Build history of the part. All positions in model axes, mm. Round coordinates to 2 decimals unless told otherwise and drop trailing zeros. Loops run counter-clockwise (first coordinate to the right, second up) from the corner with the lowest first, then second, coordinate; pieces in that order, holes last. Notation, with made-up numbers: (65, 37.25) - (70, 37.25) arc R27 ccw to (70, 65.25) - close; hole circle Ø11 at (-20, 25.5). An arc over 180 degrees is marked (long way). Put each result on its own line as item: value. Start each with the question number.
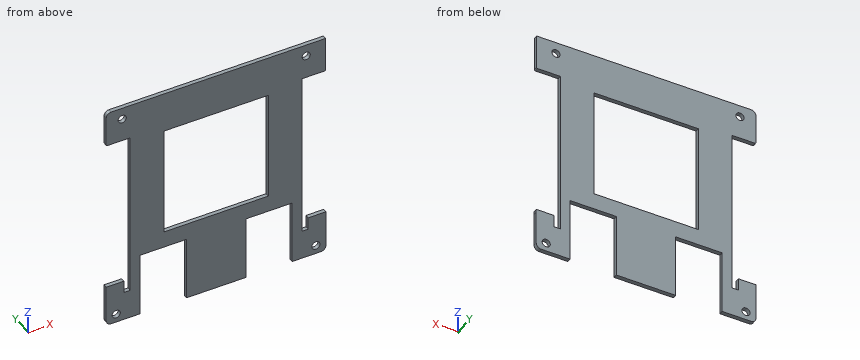
from build123d import *

# Parameters (mm, degrees)
SKETCH1_R                        = 1.6383
BOSS_EXTRUDE1_DEPTH              = 1.575
CUT_EXTRUDE1_DEPTH               = 2.54
CUTOUTS_FOR_THRUSTER_HEADS_DEPTH = 1.575
NOTCH_FOR_BPR_TOP_VIEW_W         = 2.575
NOTCH_FOR_BPR_TOP_VIEW_H         = 6.27
CUT_EXTRUDE11_DEPTH              = 10
NOTCH_FOR_BPL_TOP_VIEW_W         = 2.575
NOTCH_FOR_BPL_TOP_VIEW_H         = 6.27
CUT_EXTRUDE12_DEPTH              = 65.400936523
SKETCH22_W                       = 1.501374709
SKETCH22_H                       = 61.468
SKETCH22_W_2                     = 1.585
BOSS_EXTRUDE2_DEPTH              = 1.575
SKETCH23_W                       = 7.1002401
SKETCH23_H                       = 1.27
SKETCH23_W_2                     = 7.016
CUT_EXTRUDE13_DEPTH              = 65.400936523
SKETCH25_W                       = 2.5
SKETCH25_H                       = 44.79544
BOSS_EXTRUDE3_DEPTH              = 1.575
SKETCH26_W                       = 2.5
SKETCH26_H                       = 44.79544
BOSS_EXTRUDE4_DEPTH              = 1.575
SKETCH27_W                       = 41.818
SKETCH27_H                       = 1
CUT_EXTRUDE15_DEPTH              = 65.400936523
SKETCH28_W                       = 41.818
SKETCH28_H                       = 1
BOSS_EXTRUDE5_DEPTH              = 1.575


with BuildPart() as part:
    # Sketch1 → Boss-Extrude1 (new body)
    with BuildSketch(Plane(origin=(0, 0, 0), x_dir=(1, 0, 0), z_dir=(0, 1, 0))):
        with BuildLine():
            Line((-44, 45), (-44, 29.162404323))
            ThreePointArc((-44, 29.162404323), (-43.886381258, 28.888104416), (-43.612081351, 28.774485674))
            Line((-43.612081351, 28.774485674), (-33.211918649, 28.774485674))
            ThreePointArc((-33.211918649, 28.774485674), (-32.937618742, 28.660866933), (-32.824, 28.386567026))
            Line((-32.824, 28.386567026), (-32.824, -32.305595677))
            ThreePointArc((-32.824, -32.305595677), (-32.937618742, -32.579895584), (-33.211918649, -32.693514326))
            Line((-33.211918649, -32.693514326), (-36.100000052, -32.693514326))
            Line((-36.100000052, -32.693514326), (-43.612081299, -32.693514326))
            ThreePointArc((-43.612081299, -32.693514326), (-43.886381206, -32.807133067), (-43.999999948, -33.081432974))
            Line((-43.999999948, -33.081432974), (-43.999999948, -38.977))
            Line((-43.999999948, -38.977), (-43.999999948, -45))
            ThreePointArc((-43.999999948, -45), (-43.41421351, -46.414213562), (-41.999999948, -47))
            Line((-41.999999948, -47), (42.705916546, -47))
            Line((42.705916546, -47), (43.849731117, -47))
            Line((43.849731117, -47), (43.849731117, -38.27))
            Line((43.849731117, -38.27), (43.849731117, -33.081432974))
            ThreePointArc((43.849731117, -33.081432974), (43.736112376, -32.807133067), (43.461812469, -32.693514326))
            Line((43.461812469, -32.693514326), (36.098785193, -32.693514326))
            Line((36.098785193, -32.693514326), (33.824, -32.693514326))
            Line((33.824, -32.693514326), (32.822785141, -32.693514326))
            Line((32.822785141, -32.693514326), (32.822785141, -30.469351623))
            Line((32.822785141, -30.469351623), (32.822785141, 27.774485674))
            ThreePointArc((32.822785141, 27.774485674), (33.11567836, 28.481592456), (33.822785141, 28.774485674))
            Line((33.822785141, 28.774485674), (43.611054239, 28.774485674))
            ThreePointArc((43.611054239, 28.774485674), (43.885287743, 28.88803803), (43.998972842, 29.162216531))
            Line((43.998972842, 29.162216531), (44, 31.284))
            Line((44, 31.284), (44, 45))
            ThreePointArc((44, 45), (43.414213562, 46.414213562), (42, 47))
            Line((42, 47), (-42, 47))
            ThreePointArc((-42, 47), (-43.414213562, 46.414213562), (-44, 45))
        make_face()
        with Locations(Location((40, 43.5, 0), (0, 0, 270))):
            Circle(SKETCH1_R, mode=Mode.SUBTRACT)
        with Locations(Location((-40, 43.5, 0), (0, 0, 270))):
            Circle(SKETCH1_R, mode=Mode.SUBTRACT)
        with Locations(Location((-37.599999948, -42.2, 0), (0, 0, 270))):
            Circle(SKETCH1_R, mode=Mode.SUBTRACT)
        with Locations(Location((36.100000052, -42.2, 0), (0, 0, 270))):
            Circle(SKETCH1_R, mode=Mode.SUBTRACT)
        Polygon((23.409, -31.5), (-23.409, -31.5), (-23.409, 13.29544), (-12.909, 13.29544), (-12.909, 25.99544), (12.909, 25.99544), (12.909, 13.29544), (23.409, 13.29544), align=None, mode=Mode.SUBTRACT)
    extrude(amount=BOSS_EXTRUDE1_DEPTH)

    # Sketch2 → Cut-Extrude1 (cut)
    with BuildSketch(Plane(origin=(0, 1.575, 0), x_dir=(1, 0, 0), z_dir=(0, 1, 0))):
        Polygon((-12.909, 19.06), (-30.435, 19.06), (-30.435, 47), (30.435, 47), (30.435, 19.06), (12.909, 19.06), (12.909, 25.99544), (-12.909, 25.99544), align=None)
    extrude(amount=-CUT_EXTRUDE1_DEPTH, mode=Mode.SUBTRACT)

    # Sketch16 → Cutouts for Thruster Heads (add)
    with BuildSketch(Plane(origin=(0, 1.575, 0), x_dir=(1, 0, 0), z_dir=(0, 1, 0))):
        Polygon((12.909, 19.06), (12.909, 13.29544), (-12.909, 13.29544), (-12.909, 19.06), (-30.435, 19.06), (-30.435, 21), (-11.838888217, 21), (-11.838888217, 47), (11.909, 47), (11.909, 21), (30.435, 21), (30.435, 19.06), align=None)
    extrude(amount=-CUTOUTS_FOR_THRUSTER_HEADS_DEPTH)

    # Notch for BPR (TOP VIEW) → Cut-Extrude11 (cut)
    with BuildSketch(Plane(origin=(0, 1.575, 0), x_dir=(1, 0, 0), z_dir=(0, 1, 0))):
        with Locations((-35.6965, 31.909485674)):
            Rectangle(NOTCH_FOR_BPR_TOP_VIEW_W, NOTCH_FOR_BPR_TOP_VIEW_H)
    extrude(amount=-CUT_EXTRUDE11_DEPTH, mode=Mode.SUBTRACT)

    # Notch for BPL (TOP VIEW) → Cut-Extrude12 (cut, through all)
    with BuildSketch(Plane(origin=(0, 1.575, 0), x_dir=(1, 0, 0), z_dir=(0, 1, 0))):
        with Locations((35.61165985, 31.909485674)):
            Rectangle(NOTCH_FOR_BPL_TOP_VIEW_W, NOTCH_FOR_BPL_TOP_VIEW_H)
    extrude(amount=-CUT_EXTRUDE12_DEPTH, mode=Mode.SUBTRACT)

    # Sketch22 → Boss-Extrude2 (add)
    with BuildSketch(Plane(origin=(0, 1.575, 0), x_dir=(1, 0, 0), z_dir=(0, 1, 0))):
        with Locations((33.573472495, -1.959514326)):
            Rectangle(SKETCH22_W, SKETCH22_H)
        with Locations((-33.6165, -1.959514326)):
            Rectangle(SKETCH22_W_2, SKETCH22_H)
    extrude(amount=-BOSS_EXTRUDE2_DEPTH)

    # Sketch23 → Cut-Extrude13 (cut, through all)
    with BuildSketch(Plane(origin=(0, 1.575, 0), x_dir=(1, 0, 0), z_dir=(0, 1, 0))):
        with Locations((40.4492799, 29.409485674)):
            Rectangle(SKETCH23_W, SKETCH23_H)
        with Locations((-40.492, 29.409485674)):
            Rectangle(SKETCH23_W_2, SKETCH23_H)
    extrude(amount=-CUT_EXTRUDE13_DEPTH, mode=Mode.SUBTRACT)

    # Sketch25 → Boss-Extrude3 (add)
    with BuildSketch(Plane(origin=(0, 1.575, 0), x_dir=(1, 0, 0), z_dir=(0, 1, 0))):
        with Locations((22.159, -9.10228)):
            Rectangle(SKETCH25_W, SKETCH25_H)
    extrude(amount=-BOSS_EXTRUDE3_DEPTH)

    # Sketch26 → Boss-Extrude4 (add)
    with BuildSketch(Plane(origin=(0, 1.575, 0), x_dir=(1, 0, 0), z_dir=(0, 1, 0))):
        with Locations((-22.159, -9.10228)):
            Rectangle(SKETCH26_W, SKETCH26_H)
    extrude(amount=-BOSS_EXTRUDE4_DEPTH)

    # Sketch27 → Cut-Extrude15 (cut, through all)
    with BuildSketch(Plane(origin=(0, 1.575, 0), x_dir=(1, 0, 0), z_dir=(0, 1, 0))):
        with Locations((0, 13.79544)):
            Rectangle(SKETCH27_W, SKETCH27_H)
    extrude(amount=-CUT_EXTRUDE15_DEPTH, mode=Mode.SUBTRACT)

    # Sketch28 → Boss-Extrude5 (add)
    with BuildSketch(Plane(origin=(0, 1.575, 0), x_dir=(1, 0, 0), z_dir=(0, 1, 0))):
        with Locations((0, -31)):
            Rectangle(SKETCH28_W, SKETCH28_H)
    extrude(amount=-BOSS_EXTRUDE5_DEPTH)


solid = part.part
1) Drill centre lines: line 1 (X direction, y = 0.65, z = 42.2); line 2 (X direction, y = 1.2, z = -38) (3 decimals); line 3 (X direction, y = 0.85, z = -43.5) (3 decimals). Where is each one in solid material? Low to high. Write a range as [from, to].
2) Slice it at A-A, the plane z = 16.5. Write the cut outline in (x, y) (3 decimals), and give its area (3 significant figures).
3) Slice it at D-D, the plane x = -8. Write the cut outline in (y, z) (3 decimals).
4) Slice it at B-B, the plane x = 40. Write the cut outline in (y, z) (3 decimals).
5) Drop a flat-ended pin along its axis: pin 1 Ø3 at (x, z) = (36.1, 42.2) entering from -Y. Give the stop position or say it passes through.
6) Slice it at C-C, the plane z = -43.5. Write the cut outline in (x, y) (3 decimals).
Taken from the geometry:
1. line 1: x = [-44, -39.24], [-35.96, 34.46], [37.74, 43.85]
1. line 2: x = [-44, -30.435], [-11.839, 11.909], [30.435, 44]
1. line 3: x = [-44, -41.638], [-38.362, -30.435], [-11.839, 11.909], [30.435, 38.362], [41.638, 44]
2. outline: (-34.409, 0) - (-20.909, 0) - (-20.909, 1.575) - (-34.409, 1.575) - close; (20.909, 0) - (34.324, 0) - (34.324, 1.575) - (20.909, 1.575) - close
2. area: 42.4 mm2
3. outline: (0, -47) - (1.575, -47) - (1.575, -14.295) - (0, -14.295) - close; (0, 30.5) - (1.575, 30.5) - (1.575, 47) - (0, 47) - close
4. outline: (0, -47) - (1.575, -47) - (1.575, -45.138) - (0, -45.138) - close; (0, -41.862) - (1.575, -41.862) - (1.575, -30.044) - (0, -30.044) - close; (0, 32.694) - (1.575, 32.694) - (1.575, 47) - (0, 47) - close
5. pin 1: passes through
6. outline: (-44, 0) - (-41.638, 0) - (-41.638, 1.575) - (-44, 1.575) - close; (-38.362, 0) - (-30.435, 0) - (-30.435, 1.575) - (-38.362, 1.575) - close; (-11.839, 0) - (11.909, 0) - (11.909, 1.575) - (-11.839, 1.575) - close; (30.435, 0) - (38.362, 0) - (38.362, 1.575) - (30.435, 1.575) - close; (41.638, 0) - (44, 0) - (44, 1.575) - (41.638, 1.575) - close
